Design review of the part built by this model. Coordinates are the model's own, in mm. Face numbers are marked on the shaded views. A direction names the side the tool comes from. Coordinates: 2 decimals unless noted, no trailing zeros. Loops run counter-clockwise (first coordinate to the right, second up) from the corner with the lowest first, then second, coordinate; pieces in that order, holes last. Notation, with made-up numbers: (-34.5, 70.25) -> (11.5, 70.25) arc R28 cw to (11.5, 103.25) -> close; hole circle Ø5 at (-7, 25). An arc over 180 degrees is marked (long way). One line per item, written item: value. Start each with the question number.
1. Machinability: for the marked faces 1 and 2, which of the approach directions +Z, -Z, +X, -X, +Y, -Y give a long, thin tool a straight path to every point of the face, cutting with its end or side? Answer none if there is none.
2. Add section D-D on z = 60. Write out the cut boundary in (x, y), plus the area to 3 significant figures.
3. For probe 1 along Z at (x, y) = (-141, 31); probe 2 along X at (y, z) = (27.5, 36.5); probe 3 along Y at (x, z) = (97.5, 7), list the stretches that pass through material, from the lowest coordinate up.
4. Add section B-B on x = 0. Write out the cut boundary in (y, z), plus the area to 3 significant figures.
5. Insertion check: pin 1 (19.5 mm diameter, centred on x = 55.44, z = 55.44, fed in from +Y); pin 2 (9 mm diameter, centred on x = -55.44, z = -55.44, fed in from -Y); pin 3 (17 mm diameter, centred on y = 31, z = 60, fed in from -X). Each pin has a flat end and moves straight along its axis. Give the tip position at first contact, or say it passes through.
6. Add section C-C on y = 15. Write out the cut boundary in (x, z), plus the area to 3 significant figures.
7. Add section A-A on y = 31. Write out the cut boundary in (x, z), plus the area to 3 significant figures.
```python
from build123d import *

# Parameters (mm, degrees)
SKETCH1_W                      = 296
SKETCH1_H                      = 200
BASE_FLANGE1_DEPTH             = 8
EDGE_FLANGE1_STRIP_W           = 52
EDGE_FLANGE1_STRIP_H           = 8
EDGE_FLANGE1_STRIP_CUT_DEPTH   = 200
EDGE_FLANGE1_STRIP_2_W         = 52
EDGE_FLANGE1_STRIP_2_H         = 8
EDGE_FLANGE1_STRIP_CUT_2_DEPTH = 200
EDGE_FLANGE1_DEPTH             = 200
EDGE_FLANGE1_BEND_DEPTH        = 200
SKETCH12_R                     = 30
CUT_EXTRUDE1_DEPTH             = 10
SKETCH13_R                     = 7.5
CUT_EXTRUDE2_DEPTH             = 10
SKETCH15_R                     = 7.5
CUT_EXTRUDE3_DEPTH             = 317.733326317
MIRROR5_COPY_1_SKETCH_R        = 7.5
MIRROR5_COPY_1_DEPTH           = 10


# Sheet-metal steps are written as plain solids
with BuildPart() as part:
    # Sketch1 → Base-Flange1 (new body)
    with BuildSketch(Plane(origin=(0, 0, 0), x_dir=(1, 0, 0), z_dir=(0, 1, 0))):
        Rectangle(SKETCH1_W, SKETCH1_H)
    extrude(amount=-BASE_FLANGE1_DEPTH)

    # Edge-Flange1 strip (across the edge) → Edge-Flange1 strip cut (cut)
    with BuildSketch(Plane(origin=(-148, 0, -100), x_dir=(1, 0, 0), z_dir=(0, 0, 1))):
        with Locations((-8, -4)):
            Rectangle(EDGE_FLANGE1_STRIP_W, EDGE_FLANGE1_STRIP_H)
    extrude(amount=EDGE_FLANGE1_STRIP_CUT_DEPTH, mode=Mode.SUBTRACT)

    # Edge-Flange1 strip 2 (across the edge) → Edge-Flange1 strip cut 2 (cut)
    with BuildSketch(Plane(origin=(148, 0, 100), x_dir=(-1, 0, 0), z_dir=(0, 0, -1))):
        with Locations((-8, -4)):
            Rectangle(EDGE_FLANGE1_STRIP_2_W, EDGE_FLANGE1_STRIP_2_H)
    extrude(amount=EDGE_FLANGE1_STRIP_CUT_2_DEPTH, mode=Mode.SUBTRACT)

    # Edge-Flange1 section (across the edge) → Edge-Flange1 (add)
    with BuildSketch(Plane(origin=(-148, 0, -100), x_dir=(1, 0, 0), z_dir=(0, 0, 1))):
        with BuildLine():
            Line((0, 10), (0, 52))
            Line((0, 52), (8, 52))
            Line((8, 52), (8, 10))
            ThreePointArc((8, 10), (10.928932188, 2.928932188), (18, 0))
            Line((18, 0), (18, -8))
            ThreePointArc((18, -8), (5.272077939, -2.727922061), (0, 10))
        make_face()
    extrude(amount=EDGE_FLANGE1_DEPTH)

    # Edge-Flange1 section 2 (across the edge) → Edge-Flange1 bend (add)
    with BuildSketch(Plane(origin=(148, 0, 100), x_dir=(-1, 0, 0), z_dir=(0, 0, -1))):
        with BuildLine():
            Line((0, 10), (0, 52))
            Line((0, 52), (8, 52))
            Line((8, 52), (8, 10))
            ThreePointArc((8, 10), (10.928932188, 2.928932188), (18, 0))
            Line((18, 0), (18, -8))
            ThreePointArc((18, -8), (5.272077939, -2.727922061), (0, 10))
        make_face()
    extrude(amount=EDGE_FLANGE1_BEND_DEPTH)

    # Sketch12 → Cut-Extrude1 (cut)
    with BuildSketch(Plane(origin=(0, -8, 0), x_dir=(-1, 0, 0), z_dir=(0, -1, 0))):
        with Locations(Location((0, 0, 0), (0, 0, 90))):
            Circle(SKETCH12_R)
    extrude(amount=-CUT_EXTRUDE1_DEPTH, mode=Mode.SUBTRACT)

    # Sketch13 → Cut-Extrude2 (cut)
    with BuildSketch(Plane(origin=(0, -8, 0), x_dir=(-1, 0, 0), z_dir=(0, -1, 0))):
        with Locations(Location((55.437171645, -55.437171645, 0), (0, 0, 90))):
            Circle(SKETCH13_R)
    cut_extrude2 = extrude(amount=-CUT_EXTRUDE2_DEPTH, mode=Mode.SUBTRACT)

    # Mirror4: Cut-Extrude2 across plane
    add(cut_extrude2.mirror(Plane(origin=(0, 0, 0), x_dir=(0, 0, 1), z_dir=(1, 0, 0))), mode=Mode.SUBTRACT)

    # Sketch15 → Cut-Extrude3 (cut, through all)
    with BuildSketch(Plane.ZY.offset(148)):
        with Locations(Location((-60, 31, 0), (0, 0, 270))):
            Circle(SKETCH15_R)
    cut_extrude3 = extrude(amount=-CUT_EXTRUDE3_DEPTH, mode=Mode.SUBTRACT)

    # Mirror5: Cut-Extrude2, Cut-Extrude3 across plane
    add(cut_extrude2.mirror(Plane.XY), mode=Mode.SUBTRACT)
    add(cut_extrude3.mirror(Plane.XY), mode=Mode.SUBTRACT)

    # Mirror5 copy 1 sketch → Mirror5 copy 1 (cut)
    with BuildSketch(Plane.XZ.offset(8)):
        with Locations(Location((55.437171645, -55.437171645, 0), (0, 0, 90))):
            Circle(MIRROR5_COPY_1_SKETCH_R)
    extrude(amount=-MIRROR5_COPY_1_DEPTH, mode=Mode.SUBTRACT)


solid = part.part
```
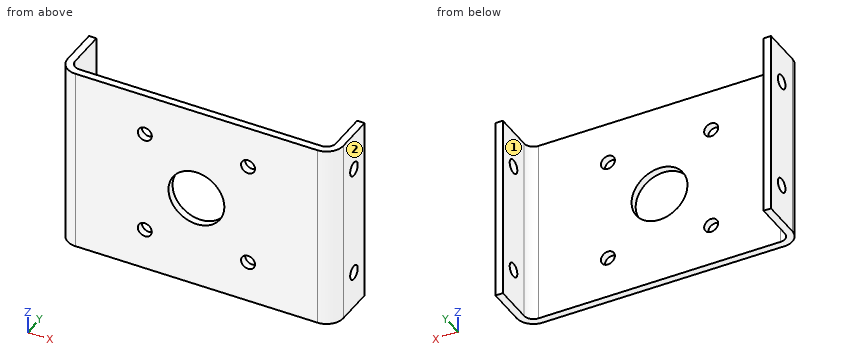
Worked answers:
1. face 1: +Z, -Z, +Y
1. face 2: +Z, -Z, +X, +Y, -Y
2. outline: (-148, 10) arc R18 ccw to (-130, -8) -> (-61.39, -8) -> (-61.39, 0) -> (-130, 0) arc R10 cw to (-140, 10) -> (-140, 23.5) -> (-148, 23.5) -> close; (-148, 38.5) -> (-140, 38.5) -> (-140, 52) -> (-148, 52) -> close; (-49.48, -8) -> (49.48, -8) -> (49.48, 0) -> (-49.48, 0) -> close; (61.39, -8) -> (130, -8) arc R18 ccw to (148, 10) -> (148, 23.5) -> (140, 23.5) -> (140, 10) arc R10 cw to (130, 0) -> (61.39, 0) -> close; (140, 38.5) -> (148, 38.5) -> (148, 52) -> (140, 52) -> close
2. area: 2,670 mm²
3. probe 1: z = -100 to -67.5, -52.5 to 52.5, 67.5 to 100
3. probe 2: x = -148 to -140, 140 to 148
3. probe 3: y = -8 to 0
4. outline: (-8, -100) -> (0, -100) -> (0, -30) -> (-8, -30) -> close; (-8, 30) -> (0, 30) -> (0, 100) -> (-8, 100) -> close
4. area: 1,120 mm²
5. pin 1: stops at y = 0
5. pin 2: passes through
5. pin 3: stops at x = -148
6. outline: (-148, -100) -> (-140, -100) -> (-140, 100) -> (-148, 100) -> close; (140, -100) -> (148, -100) -> (148, 100) -> (140, 100) -> close
6. area: 3,200 mm²
7. outline: (-148, -100) -> (-140, -100) -> (-140, -67.5) -> (-148, -67.5) -> close; (-148, -52.5) -> (-140, -52.5) -> (-140, 52.5) -> (-148, 52.5) -> close; (-148, 67.5) -> (-140, 67.5) -> (-140, 100) -> (-148, 100) -> close; (140, -100) -> (148, -100) -> (148, -67.5) -> (140, -67.5) -> close; (140, -52.5) -> (148, -52.5) -> (148, 52.5) -> (140, 52.5) -> close; (140, 67.5) -> (148, 67.5) -> (148, 100) -> (140, 100) -> close
7. area: 2,720 mm²
